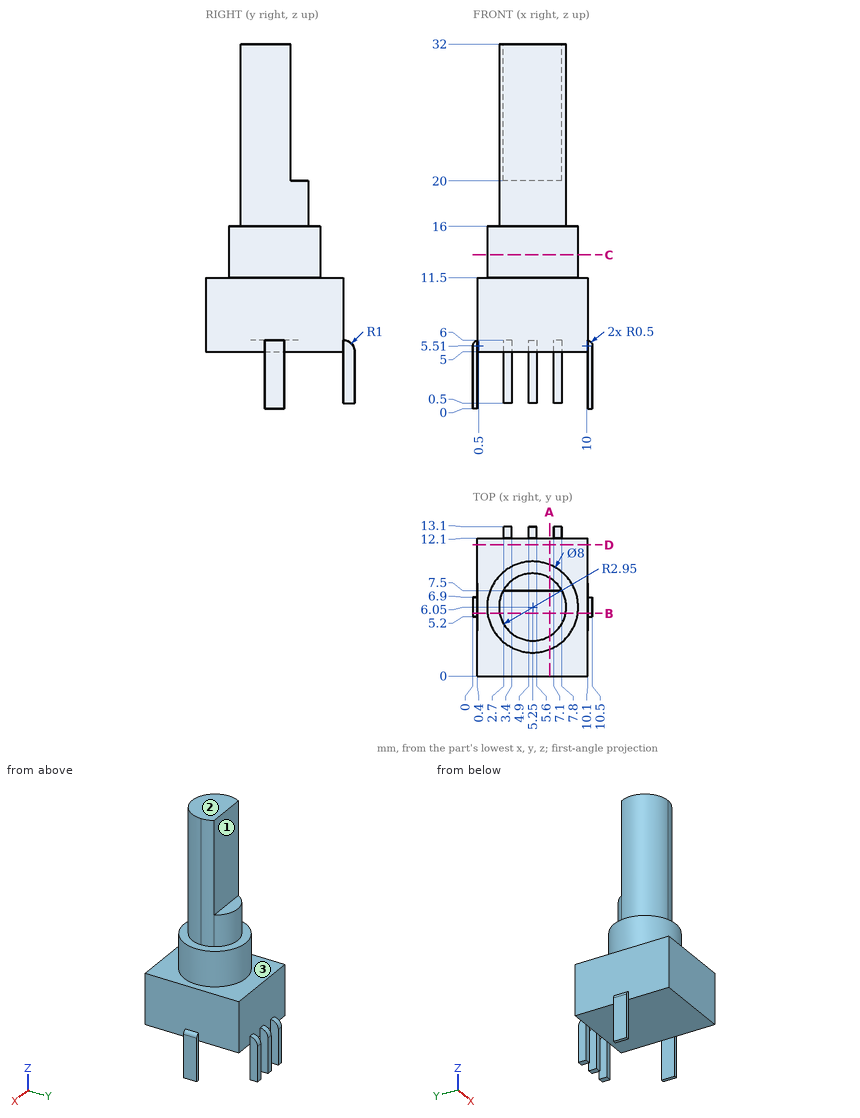
Input: dimensioned drawing with shaded views. Units: mm. Origin: part minimum x, y, z. A direction names the side the tool comes from. Give positions to 0.01 mm unless a question says otherwise; leave off trailing zeros. Write each loop counter-clockwise with the first axis right and the second up, starting at its lowest first coordinate (ties: lowest second). Pieces come first, ordered by that corner, then holes. Notation, with made-up numbers: (13.25, 69.25) -> (42.25, 69.25) arc R27 cw to (42.25, 101.25) -> close; hole circle Ø8 at (-31.5, 75). An arc over 180 degrees is marked (long way). Return JSON: item names as keys, results as strings. Group by question number.
1. Section B-B, the plane y = 5.5. Output: boundary loops of the cut face in (x, z), then the cut area to 3 significant figures.
2. Access query for the marked faces 1, 2 and 3. Directions: +Z, -Z, +X, -X, +Y, -Y. A direction counts if a zero-diameter tool reaches every point of the face in a straight line with its end or side. Return the directions, or none.
3. Section C-C, the plane z = 13.5. Output: boundary loops of the cut face in (x, y), then the cut area to 3 significant figures.
4. Material intervals for line 1 (X direction, y = 1, z = 8); line 2 (Y direction, x = 3, z = 8.5); line 3 (Z direction, x = 3, y = 1.25), sorted ascending. Write a range as from..to.
5. Section A-A, the plane x = 6.75. Output: boundary loops of the cut face in (y, z), then the cut area to 3 significant figures.
6. Section D-D, the plane y = 11.5. Output: boundary loops of the cut face in (x, z).
7. Pin query (flat end, axial travel): pin 1 Ø0.6 at (x, z) = (5, 3) entering from -Y; pin 2 Ø1.4 at (y, z) = (6, 1.5) entering from -X; pin 3 Ø1.1 at (y, z) = (12.5, 2) entering from -X; pin 4 Ø2 at (x, z) = (8, 22.5) entering from +Y. Return the tip coordinate at first contact, or that it passes through.
Determined:
{
 "1": {"outline": "(0, 0) -> (0.4, 0) -> (0.4, 5) -> (10.1, 5) -> (10.1, 0) -> (10.5, 0) -> (10.5, 5.51) arc R0.5 ccw to (10.1, 6) -> (10.1, 11.5) -> (9.21, 11.5) -> (9.21, 16) -> (8.15, 16) -> (8.15, 32) -> (2.35, 32) -> (2.35, 16) -> (1.29, 16) -> (1.29, 11.5) -> (0.4, 11.5) -> (0.4, 6) arc R0.5 ccw to (0, 5.51) -> close", "area": "196 mm2"},
 "2": {"face 1": "+Z, +X, -X, +Y", "face 2": "+Z, +X, -X, +Y, -Y", "face 3": "+Z"},
 "3": {"outline": "circle Ø8 at (5.25, 6.05)", "area": "50.3 mm2"},
 "4": {"line 1": "x = 0.4..10.1", "line 2": "y = 0..12.1", "line 3": "z = 5..11.5"},
 "5": {"outline": "(0, 5) -> (12.1, 5) -> (12.1, 11.5) -> (9.76, 11.5) -> (9.76, 16) -> (8.59, 16) -> (8.59, 20) -> (7.5, 20) -> (7.5, 32) -> (3.51, 32) -> (3.51, 16) -> (2.34, 16) -> (2.34, 11.5) -> (0, 11.5) -> close", "area": "180 mm2"},
 "6": {"outline": "(0.4, 5) -> (10.1, 5) -> (10.1, 11.5) -> (0.4, 11.5) -> close"},
 "7": {"pin 1": "stops at y = 12.1", "pin 2": "stops at x = 0", "pin 3": "stops at x = 2.7", "pin 4": "stops at y = 7.5"}
}
